Solid Edge part; units mm, degrees
sketch "Sketch1" plane through (0, 0, 0) normal (0, -1, 0) x (1, 0, 0)
  line L0 (-200, 250) -> (-200, 450)
  line L1 (-200, 450) -> (100, 450)
  line L2 (100, 450) -> (100, 250)
  line L3 (100, 250) -> (400, 250)
  line L4 (400, 250) -> (400, 0)
  line L5 (400, 0) -> (0, 0)
  line L6 (0, 0) -> (-500, 0)
  line L7 (-500, 0) -> (-500, 250)
  line L8 (-500, 250) -> (-200, 250)
revolve "RevolvedProtrusion1" add sketch "Sketch1" angle 360 about axis through (-500, 0, -125) along (1, 0, 0)
Check sheet for the modelled part. Datum: model origin and axes. Units: mm. A direction names the side the tool comes from. Coordinates: 2 decimals unless noted, no trailing zeros. Loops run counter-clockwise (first coordinate to the right, second up) from the corner with the lowest first, then second, coordinate; pieces in that order, holes last. Notation, with made-up numbers: (-9.75, 85) -> (3.25, 85) arc R21 cw to (3.25, 115) -> close; hole circle Ø5 at (45, 0.5). An arc over 180 degrees is marked (long way). Write item = value, one per line. Start each with the question number.
1. Section check C-C on x = -255.5. Record the cut outline in (y, z).
2. Tool access check on faces 1 (the flat face through (400, -89, -214)), 2 (the cylindrical face through (-347.9, -112.64, 232.683)), 3 (the flat face through (100, 375.3, -133)). Record the directions out of +Z, -Z, +X, -X, +Y, -Y that give a thin tool (end or side, any length) a straight path to the whole face; none if there is none.
3. Material ranges on line 1 (Y direction, x = 0, z = -125); line 2 (Z direction, x = -256, y = 0); line 3 (Y direction, x = -292, z = -125), recorded low to high.
4. Section check D-D on x = -8. Record the cut outline in (y, z), then the cut area to 3 significant figures.
5. Section check B-B on y = 0. Record the cut outline in (x, z).
6. Section check A-A on z = -125. Record the cut outline in (x, y), then the cut area to 3 significant figures.
7. Depth check by flat-ended pin: P1, Ø2, axis at x = 130, z = -374, coming from the +Y side; P2, Ø3, axis at x = 21, y = 115, coming from the -Z side; P3, Ø5, axis at y = -395, z = -318, coming from the -X side. Enter the tip coordinate at first touch or a pass-through.
8. Draft check along Z on faces 4 (the cylindrical face through (-56.3, 5.5, -249.88)), 5 (the flat face through (-200, 375.3, -133)), 6 (the cylindrical face through (252.1, -112.64, 232.683)). Enter one of: released by +Z, released by -Z, zero draft, split by the parting line, or undercut.
Responses:
q1.outline = circle Ø750 at (0, -125); hole circle Ø250 at (0, -125)
q2.face_1 = +Z, -Z, +X, +Y, -Y
q2.face_2 = -X
q2.face_3 = +X
q3.line_1 = -575 to -125, 125 to 575
q3.line_2 = -500 to -250, 0 to 250
q3.line_3 = -375 to -125, 125 to 375
q4.outline = circle Ø1150 at (0, -125); hole circle Ø250 at (0, -125)
q4.area = 990,000 mm2
q5.outline = (-500, -500) -> (-200, -500) -> (-200, -700) -> (100, -700) -> (100, -500) -> (400, -500) -> (400, -250) -> (-500, -250) -> close; (-500, 0) -> (400, 0) -> (400, 250) -> (100, 250) -> (100, 450) -> (-200, 450) -> (-200, 250) -> (-500, 250) -> close
q6.outline = (-500, -375) -> (-200, -375) -> (-200, -575) -> (100, -575) -> (100, -375) -> (400, -375) -> (400, -125) -> (-500, -125) -> close; (-500, 125) -> (400, 125) -> (400, 375) -> (100, 375) -> (100, 575) -> (-200, 575) -> (-200, 375) -> (-500, 375) -> close
q6.area = 570,000 mm2
q7.P1 = 281.28
q7.P2 = -688.69
q7.P3 = -200
q8.face_4 = undercut
q8.face_5 = zero draft
q8.face_6 = split by the parting line
